Geometry: final body of the model. Coordinates: model frame, mm. A direction names the side the tool comes from. Round coordinates to 2 decimals unless told otherwise and drop trailing zeros. Loops run counter-clockwise (first coordinate to the right, second up) from the corner with the lowest first, then second, coordinate; pieces in that order, holes last. Notation, with made-up numbers: (58, 25.25) - (63, 25.25) arc R25 ccw to (63, 43.25) - close; hole circle Ø11 at (50.5, 85). An arc over 180 degrees is marked (long way). Return JSON: item names as keys, results as strings. Group by question number.
1. Section D-D on y = 1.7. Count the separate pieces of the cut face and the enclosed holes in it, and give its area (3 significant figures).
2. Set-up query: faces 1 (the face through (15, 2, -1)), 2 (the face through (-23.57, 1.01, -66.94)). Return all of +Z, -Z, +X, -X, +Y, -Y with unobstructed straight access to the full face (end or side cutting, diameter ignored); none if empty.
3. Section A-A on z = 34. Return loops of the section in (x, y).
4. Section C-C on z = -70. Return loops of the section in (x, y).
5. Section B-B on x = 3.5. Return loops of the section in (y, z).
6. Material intervals for probe 1 along X at (y, z) = (0.7, 32); probe 2 along X at (y, z) = (0.9, -30); probe 3 along Z at (x, y) = (-11.5, 0.85), sorted ascending.
from build123d import *

# Parameters (mm, degrees)
SKETCH_1_W               = 180
SKETCH_1_H               = 180
EXTRUDE_1_DEPTH          = 2
SKETCH_2_R               = 1.5
CUT_EXTRUDE_1_DEPTH      = 3
SKETCH_3_W               = 28
SKETCH_3_H               = 15
SKETCH_3_W_2             = 35
SKETCH_3_W_3             = 12
SKETCH_3_H_2             = 25
CUT_EXTRUDE_2_DEPTH      = 3
FILLET_1_R               = 3
SKETCH_5_R               = 1.7
CUT_EXTRUDE_3_DEPTH      = 128.294933128
CUT_EXTRUDE_4_DEPTH      = 10
SKETCH_7_R               = 1.6
CUT_EXTRUDE_5_DEPTH      = 10
FILLET_2_R               = 3
FILLET_3_R               = 1
CUT_EXTRUDE_6_DEPTH      = 128.294933128
CUT_EXTRUDE_6_DEPTH_BACK = 128.294933128
SKETCH_8_R               = 1.6
FILLET_4_R               = 2


with BuildPart() as part:
    # 草图1 → 凸台-拉伸1 (new body)
    with BuildSketch(Plane(origin=(0, 0, 0), x_dir=(1, 0, 0), z_dir=(0, 1, 0))):
        Rectangle(SKETCH_1_W, SKETCH_1_H)
    extrude(amount=EXTRUDE_1_DEPTH)

    # 草图2 → 切除-拉伸1 (cut)
    with BuildSketch(Plane(origin=(0, 2, 0), x_dir=(1, 0, 0), z_dir=(0, 1, 0))):
        with Locations(Location((-42.9895, 66.2305, 0), (0, 0, 270))):
            Circle(SKETCH_2_R)
        with Locations(Location((42.9895, 66.2305, 0), (0, 0, 270))):
            Circle(SKETCH_2_R)
        with Locations(Location((-42.9895, -66.2305, 0), (0, 0, 270))):
            Circle(SKETCH_2_R)
        with Locations(Location((42.9895, -66.2305, 0), (0, 0, 270))):
            Circle(SKETCH_2_R)
    extrude(amount=-CUT_EXTRUDE_1_DEPTH, mode=Mode.SUBTRACT)

    # 草图3 → 切除-拉伸2 (cut)
    with BuildSketch(Plane(origin=(0, 2, 0), x_dir=(1, 0, 0), z_dir=(0, 1, 0))):
        Rectangle(SKETCH_3_W, SKETCH_3_H)
        with Locations((-25, 35)):
            Rectangle(SKETCH_3_W_2, SKETCH_3_H)
        with Locations((25, 35)):
            Rectangle(SKETCH_3_W_2, SKETCH_3_H)
        with Locations((45, 0)):
            Rectangle(SKETCH_3_W_3, SKETCH_3_H_2)
        with Locations((-45, 0)):
            Rectangle(SKETCH_3_W_3, SKETCH_3_H_2)
        with Locations((-25, -35)):
            Rectangle(SKETCH_3_W_2, SKETCH_3_H)
        with Locations((25, -35)):
            Rectangle(SKETCH_3_W_2, SKETCH_3_H)
        Polygon((-37, 75), (-12, 75), (-12, 60), align=None)
        Polygon((12, 75), (12, 60), (37, 75), align=None)
        Polygon((37, -75), (12, -75), (12, -60), align=None)
        Polygon((-12, -75), (-12, -60), (-37, -75), align=None)
    extrude(amount=-CUT_EXTRUDE_2_DEPTH, mode=Mode.SUBTRACT)

    # 圆角1
    fillet_1_edges = [part.edges().sort_by_distance(p)[0] for p in [
        (14, 1, -7.5),
        (14, 1, 7.5),
        (-14, 1, 7.5),
        (-14, 1, -7.5),
    ]]
    fillet(fillet_1_edges, radius=FILLET_1_R)

    # 草图5 → 切除-拉伸3 (cut, through all)
    with BuildSketch(Plane(origin=(0, 2, 0), x_dir=(1, 0, 0), z_dir=(0, 1, 0))):
        with Locations(Location((77.5, 69.014718626, 0), (0, 0, 270))):
            Circle(SKETCH_5_R)
        with Locations(Location((77.5, 85.985281374, 0), (0, 0, 270))):
            Circle(SKETCH_5_R)
        with Locations(Location((85.985281374, 77.5, 0), (0, 0, 270))):
            Circle(SKETCH_5_R)
        with Locations(Location((-85.985281374, 77.5, 0), (0, 0, 90))):
            Circle(SKETCH_5_R)
        with Locations(Location((-77.5, 85.985281374, 0), (0, 0, 90))):
            Circle(SKETCH_5_R)
        with Locations(Location((-77.5, -85.985281374, 0), (0, 0, 270))):
            Circle(SKETCH_5_R)
        with Locations(Location((-85.985281374, -77.5, 0), (0, 0, 270))):
            Circle(SKETCH_5_R)
        with Locations(Location((85.985281374, -77.5, 0), (0, 0, 90))):
            Circle(SKETCH_5_R)
        with Locations(Location((77.5, -85.985281374, 0), (0, 0, 90))):
            Circle(SKETCH_5_R)
        Polygon((80, 90), (90, 80), (90, 90), align=None)
        Polygon((-90, 90), (-80, 90), (-90, 80), align=None)
        Polygon((-80, -90), (-90, -80), (-90, -90), align=None)
        Polygon((90, -90), (80, -90), (90, -80), align=None)
    extrude(amount=-CUT_EXTRUDE_3_DEPTH, mode=Mode.SUBTRACT)

    # 草图6 → 切除-拉伸4 (cut)
    with BuildSketch(Plane(origin=(0, 2, 0), x_dir=(1, 0, 0), z_dir=(0, 1, 0))):
        Polygon((90, 70), (70, 50), (70, -50), (90, -70), align=None)
        Polygon((-70, -50), (-90, -70), (-90, 70), (-70, 50), align=None)
    extrude(amount=-CUT_EXTRUDE_4_DEPTH, mode=Mode.SUBTRACT)

    # 草图7 → 切除-拉伸5 (cut)
    with BuildSketch(Plane.XZ):
        with Locations(Location((-65, 30, 0), (0, 0, 270))):
            Circle(SKETCH_7_R)
        with Locations(Location((-65, 15, 0), (0, 0, 270))):
            Circle(SKETCH_7_R)
        with Locations(Location((-65, 45, 0), (0, 0, 270))):
            Circle(SKETCH_7_R)
        with Locations(Location((-45, 85, 0), (0, 0, 270))):
            Circle(SKETCH_7_R)
        with Locations(Location((-30, 85, 0), (0, 0, 270))):
            Circle(SKETCH_7_R)
        with Locations(Location((-15, 85, 0), (0, 0, 270))):
            Circle(SKETCH_7_R)
        with Locations(Location((15, 85, 0), (0, 0, 270))):
            Circle(SKETCH_7_R)
        with Locations(Location((30, 85, 0), (0, 0, 270))):
            Circle(SKETCH_7_R)
        with Locations(Location((45, 85, 0), (0, 0, 270))):
            Circle(SKETCH_7_R)
        with Locations(Location((-65, -45, 0), (0, 0, 270))):
            Circle(SKETCH_7_R)
        with Locations(Location((-65, -15, 0), (0, 0, 270))):
            Circle(SKETCH_7_R)
        with Locations(Location((-65, -30, 0), (0, 0, 270))):
            Circle(SKETCH_7_R)
        with Locations(Location((65, -30, 0), (0, 0, 270))):
            Circle(SKETCH_7_R)
        with Locations(Location((65, -15, 0), (0, 0, 270))):
            Circle(SKETCH_7_R)
        with Locations(Location((65, -45, 0), (0, 0, 270))):
            Circle(SKETCH_7_R)
        with Locations(Location((65, 45, 0), (0, 0, 270))):
            Circle(SKETCH_7_R)
        with Locations(Location((65, 15, 0), (0, 0, 270))):
            Circle(SKETCH_7_R)
        with Locations(Location((65, 30, 0), (0, 0, 270))):
            Circle(SKETCH_7_R)
        with Locations(Location((45, -85, 0), (0, 0, 270))):
            Circle(SKETCH_7_R)
        with Locations(Location((30, -85, 0), (0, 0, 270))):
            Circle(SKETCH_7_R)
        with Locations(Location((15, -85, 0), (0, 0, 270))):
            Circle(SKETCH_7_R)
        with Locations(Location((-15, -85, 0), (0, 0, 270))):
            Circle(SKETCH_7_R)
        with Locations(Location((-30, -85, 0), (0, 0, 270))):
            Circle(SKETCH_7_R)
        with Locations(Location((-45, -85, 0), (0, 0, 270))):
            Circle(SKETCH_7_R)
        with Locations(Location((-65, 85, 0), (0, 0, 270))):
            Circle(SKETCH_7_R)
        with Locations(Location((65, 85, 0), (0, 0, 270))):
            Circle(SKETCH_7_R)
        with Locations(Location((65, -85, 0), (0, 0, 270))):
            Circle(SKETCH_7_R)
        with Locations(Location((-65, -85, 0), (0, 0, 270))):
            Circle(SKETCH_7_R)
    extrude(amount=-CUT_EXTRUDE_5_DEPTH, mode=Mode.SUBTRACT)

    # 圆角2
    fillet_2_edges = [part.edges().sort_by_distance(p)[0] for p in [
        (42.5, 1, -42.5),
        (42.5, 1, -27.5),
        (7.5, 1, -27.5),
        (7.5, 1, -42.5),
        (-39, 1, -12.5),
        (-39, 1, 12.5),
        (-51, 1, 12.5),
        (-51, 1, -12.5),
        (51, 1, -12.5),
        (51, 1, 12.5),
        (39, 1, 12.5),
        (39, 1, -12.5),
        (-42.5, 1, 42.5),
        (-42.5, 1, 27.5),
        (-7.5, 1, 27.5),
        (-7.5, 1, 42.5),
        (7.5, 1, 27.5),
        (42.5, 1, 27.5),
        (42.5, 1, 42.5),
        (7.5, 1, 42.5),
        (-90, 1, -80),
        (-80, 1, -90),
        (80, 1, -90),
        (90, 1, -80),
        (90, 1, 80),
        (80, 1, 90),
        (-80, 1, 90),
        (-90, 1, 80),
        (90, 1, -70),
        (90, 1, 70),
        (70, 1, 50),
        (70, 1, -50),
        (-70, 1, -50),
        (-70, 1, 50),
        (-90, 1, 70),
        (-90, 1, -70),
        (-7.5, 1, -42.5),
        (-7.5, 1, -27.5),
        (-42.5, 1, -27.5),
        (-42.5, 1, -42.5),
    ]]
    fillet(fillet_2_edges, radius=FILLET_2_R)

    # 圆角3
    fillet_3_edges = [part.edges().sort_by_distance(p)[0] for p in [
        (-12, 1, -60),
        (-37, 1, -75),
        (-12, 1, -75),
        (12, 1, -75),
        (37, 1, -75),
        (12, 1, -60),
        (-12, 1, 75),
        (-37, 1, 75),
        (-12, 1, 60),
        (12, 1, 60),
        (37, 1, 75),
        (12, 1, 75),
    ]]
    fillet(fillet_3_edges, radius=FILLET_3_R)

    # 草图8 → 切除-拉伸6 (cut, two sides: drawn at the far end of the back side and taken through both)
    with BuildSketch(Plane(origin=(0, 2, 0), x_dir=(1, 0, 0), z_dir=(0, 1, 0)).offset(-CUT_EXTRUDE_6_DEPTH_BACK)):
        with BuildLine():
            Line((-70, 48.757359313), (-70, 90))
            Line((-70, 90), (-78.757359313, 90))
            ThreePointArc((-78.757359313, 90), (-79.90540961, 89.771638598), (-80.878679656, 89.121320344))
            Line((-80.878679656, 89.121320344), (-89.121320344, 80.878679656))
            ThreePointArc((-89.121320344, 80.878679656), (-89.771638598, 79.90540961), (-90, 78.757359313))
            Line((-90, 78.757359313), (-90, 71.242640687))
            ThreePointArc((-90, 71.242640687), (-89.771638598, 70.09459039), (-89.121320344, 69.121320344))
            Line((-89.121320344, 69.121320344), (-70.878679656, 50.878679656))
            ThreePointArc((-70.878679656, 50.878679656), (-70.228361402, 49.90540961), (-70, 48.757359313))
        make_face()
        with BuildLine():
            Line((-70, -90), (-70, -48.757359313))
            ThreePointArc((-70, -48.757359313), (-70.228361402, -49.90540961), (-70.878679656, -50.878679656))
            Line((-70.878679656, -50.878679656), (-89.121320344, -69.121320344))
            ThreePointArc((-89.121320344, -69.121320344), (-89.771638598, -70.09459039), (-90, -71.242640687))
            Line((-90, -71.242640687), (-90, -78.757359313))
            ThreePointArc((-90, -78.757359313), (-89.771638598, -79.90540961), (-89.121320344, -80.878679656))
            Line((-89.121320344, -80.878679656), (-80.878679656, -89.121320344))
            ThreePointArc((-80.878679656, -89.121320344), (-79.90540961, -89.771638598), (-78.757359313, -90))
            Line((-78.757359313, -90), (-70, -90))
        make_face()
        with BuildLine():
            ThreePointArc((70.878679656, -50.878679656), (70.228361402, -49.90540961), (70, -48.757359313))
            Line((70, -48.757359313), (70, -90))
            Line((70, -90), (78.757359313, -90))
            ThreePointArc((78.757359313, -90), (79.90540961, -89.771638598), (80.878679656, -89.121320344))
            Line((80.878679656, -89.121320344), (89.121320344, -80.878679656))
            ThreePointArc((89.121320344, -80.878679656), (89.771638598, -79.90540961), (90, -78.757359313))
            Line((90, -78.757359313), (90, -71.242640687))
            ThreePointArc((90, -71.242640687), (89.771638598, -70.09459039), (89.121320344, -69.121320344))
            Line((89.121320344, -69.121320344), (70.878679656, -50.878679656))
        make_face()
        with BuildLine():
            Line((78.757359313, 90), (70, 90))
            Line((70, 90), (70, 48.757359313))
            ThreePointArc((70, 48.757359313), (70.228361402, 49.90540961), (70.878679656, 50.878679656))
            Line((70.878679656, 50.878679656), (89.121320344, 69.121320344))
            ThreePointArc((89.121320344, 69.121320344), (89.771638598, 70.09459039), (90, 71.242640687))
            Line((90, 71.242640687), (90, 78.757359313))
            ThreePointArc((90, 78.757359313), (89.771638598, 79.90540961), (89.121320344, 80.878679656))
            Line((89.121320344, 80.878679656), (80.878679656, 89.121320344))
            ThreePointArc((80.878679656, 89.121320344), (79.90540961, 89.771638598), (78.757359313, 90))
        make_face()
        with Locations(Location((-65, 0, 0), (0, 0, 270))):
            Circle(SKETCH_8_R)
        with Locations(Location((-25, 0, 0), (0, 0, 270))):
            Circle(SKETCH_8_R)
        with Locations(Location((25, 0, 0), (0, 0, 90))):
            Circle(SKETCH_8_R)
        with Locations(Location((65, 0, 0), (0, 0, 90))):
            Circle(SKETCH_8_R)
    extrude(amount=CUT_EXTRUDE_6_DEPTH + CUT_EXTRUDE_6_DEPTH_BACK, mode=Mode.SUBTRACT)

    # 圆角4
    fillet_4_edges = [part.edges().sort_by_distance(p)[0] for p in [
        (-70, 1, 90),
        (70, 1, 90),
        (70, 1, -90),
        (-70, 1, -90),
    ]]
    fillet(fillet_4_edges, radius=FILLET_4_R)


solid = part.part
Taken from the geometry:
{
 "1": {"separate pieces": "1", "enclosed holes": "47", "area": "21,100 mm2"},
 "2": {"face 1": "+Z, -Z, +X, -X, +Y", "face 2": "+Y, -Y"},
 "3": {"outline": "(-70, 0) - (-42.5, 0) - (-42.5, 2) - (-70, 2) - close; (-7.5, 0) - (7.5, 0) - (7.5, 2) - (-7.5, 2) - close; (42.5, 0) - (70, 0) - (70, 2) - (42.5, 2) - close"},
 "4": {"outline": "(-70, 0) - (-28.67, 0) - (-28.67, 2) - (-70, 2) - close; (-12, 0) - (12, 0) - (12, 2) - (-12, 2) - close; (28.67, 0) - (70, 0) - (70, 2) - (28.67, 2) - close"},
 "5": {"outline": "(0, -90) - (2, -90) - (2, -7.5) - (0, -7.5) - close; (0, 7.5) - (2, 7.5) - (2, 90) - (0, 90) - close"},
 "6": {"probe 1": "-70 to -42.5, -7.5 to 7.5, 42.5 to 70", "probe 2": "-70 to -66.6, -63.4 to -42.46, -7.54 to 7.54, 42.46 to 63.4, 66.6 to 70", "probe 3": "-90 to -42.5, -27.5 to -7.46, 7.46 to 27.5, 42.5 to 90"}
}
